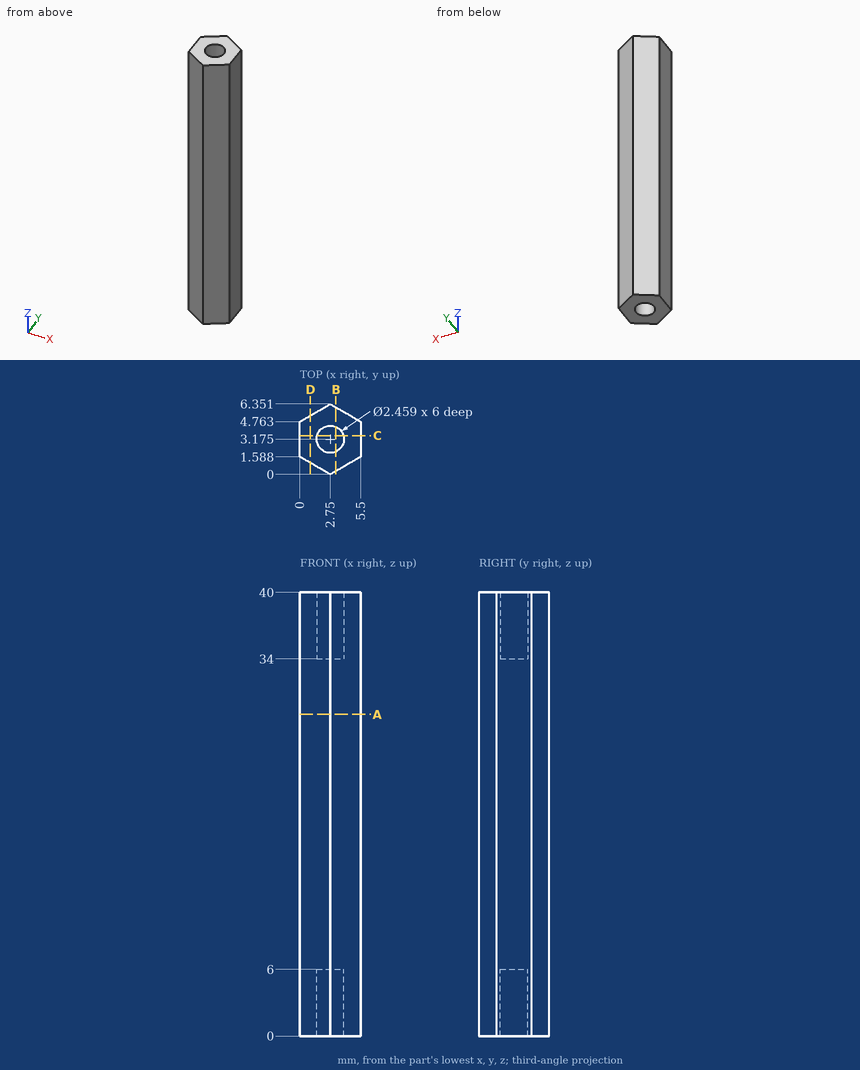
Could you check a few things on this drawing? It's one solid part, dimensions in mm from its lowest x, y, z. Round coordinates to 2 decimals unless told otherwise and drop trailing zeros. Write each loop counter-clockwise with the first axis right and the second up, starting at its lowest first coordinate (ties: lowest second). Pieces come first, ordered by that corner, then holes. Notation, with made-up numbers: M 59,-27.75 L 81,-27.75 A15 cw 81,-8.75 Z; hole C 49,36.5 d6. An arc over 180 degrees is marked long. Answer as CSV lines item,"result". Start each with the question number.
1. Suppose I cut it at D-D on x = 0.95. Write out the boundary of the cut face in (y, z).
2. Suppose I cut it at B-B on x = 3.25. Write out the boundary of the cut face in (y, z), then the cut area to 3 significant figures.
3. Suppose I cut it at C-C on y = 3.5. Write out the boundary of the cut face in (x, z).
4. Suppose I cut it at A-A on z = 29. Write out the boundary of the cut face in (x, y), then the cut area to 3 significant figures.
5. I need wall thicknesses on probe 1 along X at (y, z) = (5.5, 35) (1 decimal); probe 2 along Y at (x, z) = (4.2, 6) (1 decimal); probe 3 along Y at (x, z) = (2.1, 20.5) (1 decimal). Which ranges of each line are inside material? Lowest first, please.
6. I'm going to push flat-ended pins straight in: pin 1 Ø1.5 at (x, y) = (2.75, 3.18) entering from -Z; pin 2 Ø2.5 at (x, y) = (2.5, 3) entering from -Z; pin 3 Ø2 at (x, z) = (0.5, 8) entering from -Y; pin 4 Ø2 at (x, y) = (2.75, 3.18) entering from +Z. Where does each tip first touch, or does it pass through?
Check result:
1,outline,"M 1.04,0 L 5.31,0 L 5.31,40 L 1.04,40 Z"
2,outline,"M 0.29,0 L 2.05,0 L 2.05,6 L 4.3,6 L 4.3,0 L 6.06,0 L 6.06,40 L 4.3,40 L 4.3,34 L 2.05,34 L 2.05,40 L 0.29,40 Z"
2,area,"204 mm2"
3,outline,"M 0,0 L 1.56,0 L 1.56,6 L 3.94,6 L 3.94,0 L 5.5,0 L 5.5,40 L 3.94,40 L 3.94,34 L 1.56,34 L 1.56,40 L 0,40 Z"
4,outline,"M 0,1.59 L 2.75,0 L 5.5,1.59 L 5.5,4.76 L 2.75,6.35 L 0,4.76 Z"
4,area,"26.2 mm2"
5,probe 1,"x = 1.3 to 4.2"
5,probe 2,"y = 0.8 to 5.5"
5,probe 3,"y = 0.4 to 6"
6,pin 1,"stops at z = 6"
6,pin 2,"stops at z = 0"
6,pin 3,"stops at y = 0.72"
6,pin 4,"stops at z = 34"
